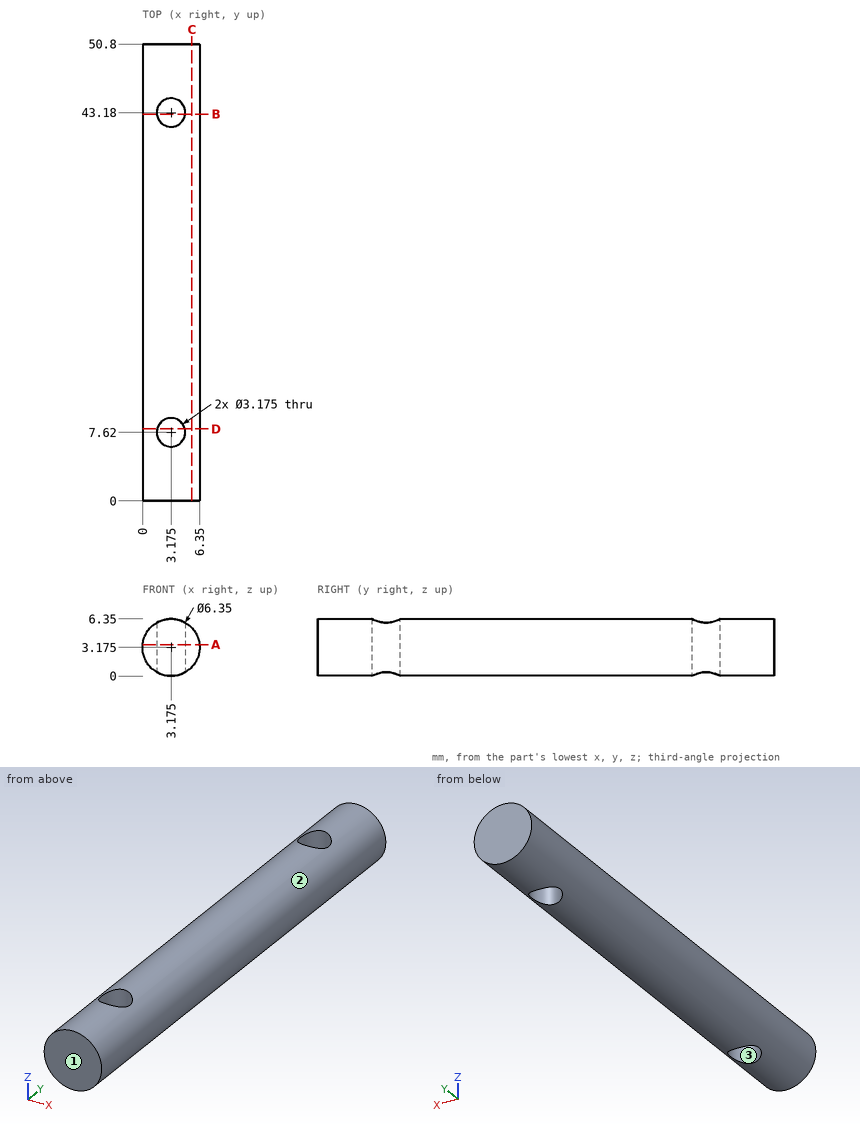
Design review of the part shown in the three views and the two pictorial views. Dimensions are in mm from the part's minimum x, y and z. Round coordinates to 2 decimals unless told otherwise and drop trailing zeros. Loops run counter-clockwise (first coordinate to the right, second up) from the corner with the lowest first, then second, coordinate; pieces in that order, holes last. Notation, with made-up numbers: M -37,81 L -12,81 A25 ccw -12,93 Z; hole C -12.5,81 d4. An arc over 180 degrees is marked long. Answer as a JSON object with one key per item and string values.
Item 1: We need section B-B on y = 43. Give the boundary of the cut face in (x, z) (3 decimals), and give its area (3 significant figures).
Answer sheet:
{"outline": "M 1.598,0.419 L 1.598,5.931 A3.175 ccw Z; M 4.752,0.419 A3.175 ccw 4.752,5.931 Z", "area": "12.5 mm^2"}
Item 2: We need section C-C on x = 5.5. Give the boundary of the cut face in (y, z).
Answer sheet:
{"outline": "M 0,1.01 L 50.8,1.01 L 50.8,5.34 L 0,5.34 Z"}
Item 3: We need section A-A on z = 3.5. Give the boundary of the cut face in (x, y) (1 decimal).
Answer sheet:
{"outline": "M 0,0 L 6.3,0 L 6.3,50.8 L 0,50.8 Z; hole C 3.2,7.6 d3.2; hole C 3.2,43.2 d3.2"}
Item 4: Clearance check with flat-ended pins moving along their axes: P1, Ø1, axis at x = 0.5, y = 23, coming from the +Z side; P2, Ø1.5, axis at x = 1, y = 25.5, coming from the +Z side. State where each tip first meets the part, or that it passes through.
Answer sheet:
{"P1": "stops at z = 5.49", "P2": "stops at z = 6.01"}
Item 5: We need section D-D on y = 8. Give the boundary of the cut face in (x, z) (3 decimals), and give its area (3 significant figures).
Answer sheet:
{"outline": "M 1.634,0.399 L 1.634,5.951 A3.175 ccw Z; M 4.716,0.399 A3.175 ccw 4.716,5.951 Z", "area": "12.9 mm^2"}
Item 6: Wall thickness on L1, parallel to Y at x = 3, z = 4.75; L2, parallel to X at y = 7.62, z = 3.25; L3, parallel to Y at x = 2.5, z = 3.25: over which ranges is each line inside the solid? List them lowest first. Write a range as from..to.
Answer sheet:
{"L1": "y = 0..6.04, 9.2..41.6, 44.76..50.8", "L2": "x = 0..1.59, 4.76..6.35", "L3": "y = 0..6.18, 9.06..41.74, 44.62..50.8"}
Item 7: The part is to be moulded in two halves that separate along X. For the marked faces 1, 2 and 3, say which applies: pulls with the +X half, pulls with the -X half, needs draft (parallel to the pull), parting line crosses it, or undercut.
Answer sheet:
{"face 1": "needs draft", "face 2": "parting line crosses it", "face 3": "undercut"}
